```python
from build123d import *

# Parameters (mm, degrees)
SKETCH1_R           = 2
BOSS_EXTRUDE1_DEPTH = 67
CUT_EXTRUDE1_REACH  = 30.5
CUT_EXTRUDE2_REACH  = 28.5
SKETCH3_W           = 59
SKETCH3_H           = 9.6
SKETCH4_OUTSIDE_W   = 45.996
SKETCH4_OUTSIDE_H   = 43.996
CUT_EXTRUDE3_DEPTH  = 68


with BuildPart() as part:
    # Sketch1 → Boss-Extrude1 (new body)
    with BuildSketch(Plane(origin=(0, 0, 0), x_dir=(0, 0, -1), z_dir=(1, 0, 0))):
        with BuildLine():
            Line((11.9, 1.9), (11.9, 0))
            Line((11.9, 0), (0, 0))
            Line((0, 0), (18.5, 18.5))
            Line((18.5, 18.5), (18.5, 21.5))
            ThreePointArc((18.5, 21.5), (23.5, 26.5), (28.5, 21.5))
            Line((28.5, 21.5), (28.5, 18.5))
            Line((28.5, 18.5), (11.9, 1.9))
        make_face()
        with Locations((23.5, 21.5)):
            Circle(SKETCH1_R, mode=Mode.SUBTRACT)
    extrude(amount=BOSS_EXTRUDE1_DEPTH)

    # Sketch2 → Cut-Extrude1 (cut, up to next)
    with BuildSketch(Plane(origin=(0, 0, -28.5), x_dir=(-1, 0, 0), z_dir=(0, 0, -1)), mode=Mode.PRIVATE) as cut_extrude1_sk1:
        with BuildLine():
            Line((-63, 26.5), (-63, 11.5))
            ThreePointArc((-63, 11.5), (-61.828427125, 8.671572875), (-59, 7.5))
            Line((-59, 7.5), (-8, 7.5))
            ThreePointArc((-8, 7.5), (-5.171572875, 8.671572875), (-4, 11.5))
            Line((-4, 11.5), (-4, 26.5))
            Line((-4, 26.5), (-63, 26.5))
        make_face()
    cut_extrude1_tool1 = extrude(cut_extrude1_sk1.sketch, amount=-CUT_EXTRUDE1_REACH, mode=Mode.PRIVATE) & part.part
    add(cut_extrude1_tool1.solids().sort_by_distance((33.5, 17.053049, -28.5))[0], mode=Mode.SUBTRACT)

    # Sketch3 → Cut-Extrude2 (cut, up to next)
    with BuildSketch(Plane.XZ, mode=Mode.PRIVATE) as cut_extrude2_sk1:
        with Locations((33.5, -16.7)):
            Rectangle(SKETCH3_W, SKETCH3_H)
    cut_extrude2_tool1 = extrude(cut_extrude2_sk1.sketch, amount=-CUT_EXTRUDE2_REACH, mode=Mode.PRIVATE) & part.part
    add(cut_extrude2_tool1.solids().sort_by_distance((33.5, 0, -16.7))[0], mode=Mode.SUBTRACT)

    # Sketch4 outside → Cut-Extrude3 (cut, through all)
    with BuildSketch(Plane(origin=(67, 0, 0), x_dir=(0, 0, -1), z_dir=(1, 0, 0))):
        with Locations((14.25, 13.25)):
            Rectangle(SKETCH4_OUTSIDE_W, SKETCH4_OUTSIDE_H)
        Polygon((26.396638245, 30.538773869), (-4.319805153, -0.17766953), (2.751262658, -7.248737342), (33.467706057, 23.467706057), align=None, mode=Mode.SUBTRACT)
    extrude(amount=-CUT_EXTRUDE3_DEPTH, mode=Mode.SUBTRACT)


solid = part.part
```
CAD build for the part. Positions are in the model's coordinates, mm. A direction names the side the tool comes from. Coordinates: 2 decimals unless noted, no trailing zeros. Write each loop counter-clockwise with the first axis right and the second up, starting at its lowest first coordinate (ties: lowest second). Pieces come first, ordered by that corner, then holes. Notation, with made-up numbers: (13.5, -18) -> (40.5, -18) arc R20 cw to (40.5, 12) -> close; hole circle Ø7 at (-24, -22). An arc over 180 degrees is marked (long way). Return JSON: item names as keys, results as strings. Group by question number.
Q1. Cut at C-C, the plane z = -14.75. Give the cut face in (x, y), then the cut area to 3 significant figures.
Q2. Cut at A-A, the plane z = -23.5. Give the cut face in (x, y), then the cut area to 3 significant figures.
Q3. Cut at D-D, the plane x = 18. Give the cut face in (y, z), then the cut area to 3 significant figures.
Q4. Which spindle directions (+Z, -Z, +X, -X, +Y, -Y) get a long thin tool onto all of the face, cutting with end or side? Do faces 4 (the face through (2, 20, -18.5)), 5 (the face through (61.33, 8.25, -10.22)), 6 (the face through (1.972, 21.588, -21.502)). Say none if no direction does.
Q5. Drill centre lines: line 1 (Z direction, x = 0.85, y = 21.5); line 2 (X direction, y = 7, z = -13.75); line 3 (Y direction, x = 65.85, z = -23.5). Where is each one in solid material? Low to high.
Q6. Cut at B-B, the plane y = 12.75. Give the cut face in (x, z).
Q7. Pull direction X, two halves, no side cores. Call faces 1 (the face through (1.972, 22.156, -18.543)), 2 (the face through (63, 14, -20)), 3 (the face through (67, 13, -16)): released by +X, released by -X, zero draft, split by the parting line, or undercut.
Q8. Flat gauge pins, fed straight in: pin 1 (12 mm diameter, centred on y = 18.5, z = -21, fed in from -X); pin 2 (2.5 mm diameter, centred on x = 65.5, y = 20, fed in from +Z); pin 3 (8 mm diameter, centred on x = 35.5, y = 4.5, fed in from -Z); pin 4 (4 mm diameter, centred on x = 10, z = -14.5, fed in from +Y). Where does each tip first touch, or does it go through?
Returned:
{
 "1": {"outline": "(0, 4.75) -> (4, 4.75) -> (4, 14.75) -> (0, 14.75) -> close; (63, 4.75) -> (67, 4.75) -> (67, 14.75) -> (63, 14.75) -> close", "area": "80.0 mm2"},
 "2": {"outline": "(0, 13.5) -> (4, 13.5) -> (4, 19.5) -> (0, 19.5) -> close; (0, 23.5) -> (4, 23.5) -> (4, 26.5) -> (0, 26.5) -> close; (63, 13.5) -> (67, 13.5) -> (67, 19.5) -> (63, 19.5) -> close; (63, 23.5) -> (67, 23.5) -> (67, 26.5) -> (63, 26.5) -> close", "area": "72.0 mm2"},
 "3": {"outline": "(0, -10) -> (1.9, -11.9) -> (7.5, -11.9) -> (7.5, -7.5) -> (0, 0) -> close", "area": "59.3 mm2"},
 "4": {"face 4": "+Z, +X, -X, +Y", "face 5": "+Z, -Z, +Y", "face 6": "+X, -X"},
 "5": {"line 1": "z = -28.5 to -25.5, -21.5 to -18.5", "line 2": "x = 0 to 4, 63 to 67", "line 3": "y = 13.5 to 19.5, 23.5 to 26.5"},
 "6": {"outline": "(0, -22.75) -> (4, -22.75) -> (4, -12.75) -> (0, -12.75) -> close; (63, -22.75) -> (67, -22.75) -> (67, -12.75) -> (63, -12.75) -> close"},
 "7": {"face 1": "zero draft", "face 2": "undercut", "face 3": "released by +X"},
 "8": {"pin 1": "stops at x = 0", "pin 2": "stops at z = -18.5", "pin 3": "stops at z = -11.9", "pin 4": "passes through"}
}
